For this review, take the finished solid that the model builds, in its own axes (mm). A direction names the side the tool comes from. Give positions to 0.01 mm unless a question says otherwise; leave off trailing zeros. Write each loop counter-clockwise with the first axis right and the second up, starting at its lowest first coordinate (ties: lowest second). Pieces come first, ordered by that corner, then holes. Notation, with made-up numbers: (12.25, 74.5) -> (26.25, 74.5) arc R27 cw to (26.25, 104.5) -> close; hole circle Ø5 at (47.25, -6). An arc over 180 degrees is marked (long way). Answer as CSV lines item,"result".
```python
from build123d import *

# Parameters (mm, degrees)
F1_DEPTH = 380
F2_R     = 2.5
F3_DEPTH = 25
F4_R     = 2.5
F5_DEPTH = 25


with BuildPart() as f1:
    # F0 (on Top) → F1 (new body)
    with BuildSketch(Plane.XY):
        Polygon((0, 7), (0, 0), (7, 0), (7, 5.5), (13, 5.5), (13, 0), (20, 0), (20, 7), (14.5, 7), (14.5, 13), (20, 13), (20, 20), (13, 20), (13, 14.5), (7, 14.5), (7, 20), (0, 20), (0, 13), (5.5, 13), (5.5, 7), align=None)
    extrude(amount=F1_DEPTH)

    # F2 (on face) → F3 (cut)
    with BuildSketch(Plane.YZ.offset(14.5)):
        with Locations((10, 70)):
            Circle(F2_R)
    extrude(amount=-F3_DEPTH, mode=Mode.SUBTRACT)

    # F4 (on face) → F5 (cut)
    with BuildSketch(Plane.XZ.offset(-5.5)):
        with Locations((10, 70)):
            Circle(F4_R)
    extrude(amount=-F5_DEPTH, mode=Mode.SUBTRACT)


solid = f1.part
```
Q1. Clearance check with flat-ended pins moving along their axes: pin 1 (3 mm diameter, centred on y = 10, z = 297, fed in from +X); pin 2 (3 mm diameter, centred on x = 10, z = 113.5, fed in from +Y). State where each tip first meets the part, or that it passes through.
Answer block:
pin 1,"stops at x = 14.5"
pin 2,"stops at y = 14.5"
Q2. To check wall thickness, follow probe 1 along Z at (x, y) = (7.6, 10); probe 2 along Y at (x, z) = (4.25, 243). State the ranges of each line that lie inside material, in increasing order. Write a range as [from, to].
Answer block:
probe 1,"z = [0, 67.5], [72.5, 380]"
probe 2,"y = [0, 7], [13, 20]"
Q3. Add section A-A (z = 318). Write out the cut boundary in (x, y), plus the area to 3 significant figures.
Answer block:
outline,"(0, 0) -> (7, 0) -> (7, 5.5) -> (13, 5.5) -> (13, 0) -> (20, 0) -> (20, 7) -> (14.5, 7) -> (14.5, 13) -> (20, 13) -> (20, 20) -> (13, 20) -> (13, 14.5) -> (7, 14.5) -> (7, 20) -> (0, 20) -> (0, 13) -> (5.5, 13) -> (5.5, 7) -> (0, 7) -> close"
area,"268 mm2"
Q4. Draft analysis for pull direction Y (two halves, no side actions). For faces 1 (the flat face through (5.5, 10, 187)), 2 (the flat face through (14.5, 10, 187)), 3 (the flat face through (10, 14.5, 187)), 4 (the flat face through (10, 10, 380)), state which applies: released by +Y, released by -Y, zero draft, split by the parting line, or undercut.
Answer block:
face 1,"undercut"
face 2,"undercut"
face 3,"released by +Y"
face 4,"zero draft"
Q5. For faces 5 (the flat face through (17, 20, 187)), 6 (the flat face through (10, 5.5, 187)), list the 3-axis set-ups (+Z, -Z, +X, -X, +Y, -Y) from which the entire face can be reached by the end or side of a thin tool; tool diameter is ignored.
Answer block:
face 5,"+Z, -Z, +X, -X, +Y"
face 6,"+Z, -Z, -Y"
